Verification items for the finished model (mm, model axes). A direction names the side the tool comes from. Give positions to 0.01 mm unless a question says otherwise; leave off trailing zeros. Order: outer loops, then holes, each group sorted by start corner. A loop starts at its lowest first (then second) coordinate and runs counter-clockwise, first axis right, second up.
from build123d import *

# Parameters (mm, degrees)
CROQUIS1_R              = 7.5
SALIENTE_EXTRUIR1_DEPTH = 10
SALIENTE_EXTRUIR2_DEPTH = 80
CORTAR_EXTRUIR1_DEPTH   = 50
CROQUIS5_R              = 10
CORTAR_EXTRUIR2_DEPTH   = 50
CORTAR_EXTRUIR3_DEPTH   = 50


with BuildPart() as part:
    # Croquis1 → Saliente-Extruir1 (new body)
    with BuildSketch(Plane(origin=(0, 0, 0), x_dir=(1, 0, 0), z_dir=(0, 1, 0))):
        with BuildLine():
            Line((-6.338028169, 29.322847729), (-74.169014085, 14.661423864))
            ThreePointArc((-74.169014085, 14.661423864), (-86, 0), (-74.169014085, -14.661423864))
            Line((-74.169014085, -14.661423864), (-6.338028169, -29.322847729))
            ThreePointArc((-6.338028169, -29.322847729), (0, -30), (6.338028169, -29.322847729))
            Line((6.338028169, -29.322847729), (74.169014085, -14.661423864))
            ThreePointArc((74.169014085, -14.661423864), (86, 0), (74.169014085, 14.661423864))
            Line((74.169014085, 14.661423864), (6.338028169, 29.322847729))
            ThreePointArc((6.338028169, 29.322847729), (0, 30), (-6.338028169, 29.322847729))
        make_face()
        with Locations((-71, 0)):
            Circle(CROQUIS1_R, mode=Mode.SUBTRACT)
        with Locations((71, 0)):
            Circle(CROQUIS1_R, mode=Mode.SUBTRACT)
    extrude(amount=SALIENTE_EXTRUIR1_DEPTH)

    # Croquis2 → Saliente-Extruir2 (add)
    with BuildSketch(Plane(origin=(0, 10, 0), x_dir=(1, 0, 0), z_dir=(0, 1, 0))):
        with BuildLine():
            Line((29.047375097, -7.5), (-29.047375097, -7.5))
            ThreePointArc((-29.047375097, -7.5), (-20.786795371, -21.631207506), (-6.338028169, -29.322847729))
            ThreePointArc((-6.338028169, -29.322847729), (0, -30), (6.338028169, -29.322847729))
            ThreePointArc((6.338028169, -29.322847729), (20.786795371, -21.631207506), (29.047375097, -7.5))
        make_face()
        with BuildLine():
            ThreePointArc((-6.338028169, 29.322847729), (-20.786795371, 21.631207506), (-29.047375097, 7.5))
            Line((-29.047375097, 7.5), (29.047375097, 7.5))
            ThreePointArc((29.047375097, 7.5), (20.786795371, 21.631207506), (6.338028169, 29.322847729))
            ThreePointArc((6.338028169, 29.322847729), (0, 30), (-6.338028169, 29.322847729))
        make_face()
    extrude(amount=SALIENTE_EXTRUIR2_DEPTH)

    # Croquis4 → Cortar-Extruir1 (cut)
    with BuildSketch(Plane(origin=(0, 90, 0), x_dir=(1, 0, 0), z_dir=(0, 1, 0))):
        with BuildLine():
            Line((-23.616731357, 18.5), (23.616731357, 18.5))
            ThreePointArc((23.616731357, 18.5), (0, 30), (-23.616731357, 18.5))
        make_face()
    extrude(amount=-CORTAR_EXTRUIR1_DEPTH, mode=Mode.SUBTRACT)

    # Croquis5 → Cortar-Extruir2 (cut)
    with BuildSketch(Plane(origin=(0, 0, -18.5), x_dir=(-1, 0, 0), z_dir=(0, 0, -1))):
        with Locations((0, 66)):
            Circle(CROQUIS5_R)
    extrude(amount=-CORTAR_EXTRUIR2_DEPTH, mode=Mode.SUBTRACT)

    # Croquis6 → Cortar-Extruir3 (cut)
    with BuildSketch(Plane(origin=(0, 90, 0), x_dir=(1, 0, 0), z_dir=(0, 1, 0))):
        with BuildLine():
            Line((-24.57931818, -17.200497604), (24.57931818, -17.200497604))
            ThreePointArc((24.57931818, -17.200497604), (0, -30), (-24.57931818, -17.200497604))
        make_face()
    extrude(amount=-CORTAR_EXTRUIR3_DEPTH, mode=Mode.SUBTRACT)


solid = part.part
(1) Section check A-A, the plane z = 0. Enter the section's corners in (x, y).
Solved:
outline: (-86, 0) - (-78.5, 0) - (-78.5, 10) - (-86, 10) - close; (-63.5, 0) - (63.5, 0) - (63.5, 10) - (-63.5, 10) - close; (78.5, 0) - (86, 0) - (86, 10) - (78.5, 10) - close
(2) Section check B-B, the plane x = -71. Enter the section's corners in (y, z), then the cut area to 3 significant figures.
Solved:
outline: (0, -15.35) - (10, -15.35) - (10, -7.5) - (0, -7.5) - close; (0, 7.5) - (10, 7.5) - (10, 15.35) - (0, 15.35) - close
area: 157 mm2
(3) Go/stop test with flat-tipped pins: pin 1 (5 mm diameter, centred on x = -26.5, y = 76.5, fed in from -Z); pin 2 (2 mm diameter, centred on y = 64.5, z = 8, fed in from -X); pin 3 (3.5 mm diameter, centred on x = 8, z = -25.5, fed in from +Y). Record where each tip stops, or that it passes through.
Solved:
pin 1: stops at z = -18
pin 2: stops at x = -29.05
pin 3: stops at y = 40
(4) Scan lines: line 1 (X direction, y = 5.5, z = 0); line 2 (Y direction, x = 0, z = 12); line 3 (Z direction, x = 23.5, y = 78). Record each from-to range of solid material in increasing order.
Solved:
line 1: x = -86 to -78.5, -63.5 to 63.5, 78.5 to 86
line 2: y = 0 to 56, 76 to 90
line 3: z = -18.5 to -7.5, 7.5 to 17.2
(5) Section check C-C, the plane y = 15.5. Enter the section's corners in (x, z).
Solved:
outline: (-29.05, -7.5) arc R30 ccw to (29.05, -7.5) - close; (-29.05, 7.5) - (29.05, 7.5) arc R30 ccw to start
(6) Set-up check for faces 1 (the flat face through (0, 49, -7.5)), 2 (the flat face through (11, 65, 17.2)), 3 (the flat face through (0, 40, -23)), 4 (the flat face through (-1, 10, 0)): record each of +Z, -Z, +X, -X, +Y, -Y from which the full face is reachable in a straight line by a thin tool's end or side.
Solved:
face 1: +X, -X, +Y
face 2: +Z, +X, -X, +Y
face 3: -Z, +X, -X, +Y
face 4: +Y
(7) Section check D-D, the plane y = 62.5. Enter the section's corners in (x, z).
Solved:
outline: (-29.05, -7.5) arc R30 ccw to (-23.62, -18.5) - (-9.37, -18.5) - (-9.37, -7.5) - close; (-29.05, 7.5) - (-9.37, 7.5) - (-9.37, 17.2) - (-24.58, 17.2) arc R30 ccw to start; (9.37, -18.5) - (23.62, -18.5) arc R30 ccw to (29.05, -7.5) - (9.37, -7.5) - close; (9.37, 7.5) - (29.05, 7.5) arc R30 ccw to (24.58, 17.2) - (9.37, 17.2) - close
(8) Release check for a two-part mould opening along X. For faces 5 (the flat face through (40.73, 4.93, -21.89)), 6 (the cylindrical face through (63.507, 4.93, -0.33)), 7 (the flat face through (0, 90, -13)), 8 (the cylindrical face through (-78.493, 4.93, -0.33)) record: pulls with the +X half, pulls with the -X half, needs draft (parallel to the pull), parting line crosses it, or undercut.
Solved:
face 5: pulls with the +X half
face 6: undercut
face 7: needs draft
face 8: undercut
